```python
from build123d import *

# Parameters (mm, degrees)
SKETCH_4_R      = 1
EXTRUDE_1_DEPTH = 3


with BuildPart() as part:
    # ｽｹｯﾁ4 → ﾎﾞｽ - 押し出し1 (new body)
    with BuildSketch(Plane(origin=(0, 0, 0), x_dir=(1, 0, 0), z_dir=(0, 1, 0))):
        with BuildLine():
            Line((13.643014387, 25.949889929), (-16.356985613, 25.949889929))
            ThreePointArc((-16.356985613, 25.949889929), (-23.428053425, 23.020957741), (-26.356985613, 15.949889929))
            Line((-26.356985613, 15.949889929), (-26.356985613, -14.050110071))
            ThreePointArc((-26.356985613, -14.050110071), (-23.428053425, -21.121177883), (-16.356985613, -24.050110071))
            Line((-16.356985613, -24.050110071), (13.643014387, -24.050110071))
            ThreePointArc((13.643014387, -24.050110071), (20.714082199, -21.121177883), (23.643014387, -14.050110071))
            Line((23.643014387, -14.050110071), (23.643014387, 15.949889929))
            ThreePointArc((23.643014387, 15.949889929), (20.714082199, 23.020957741), (13.643014387, 25.949889929))
        make_face()
        with Locations(Location((16.643014387, -17.050110071, 0), (0, 0, 270))):
            Circle(SKETCH_4_R, mode=Mode.SUBTRACT)
        with Locations(Location((16.643014387, 18.949889929, 0), (0, 0, 270))):
            Circle(SKETCH_4_R, mode=Mode.SUBTRACT)
        with Locations(Location((-19.356985613, 18.949889929, 0), (0, 0, 270))):
            Circle(SKETCH_4_R, mode=Mode.SUBTRACT)
        with Locations(Location((-19.356985613, -17.050110071, 0), (0, 0, 270))):
            Circle(SKETCH_4_R, mode=Mode.SUBTRACT)
        with Locations(Location((-1.356985613, 0.949889929, 0), (0, 0, 270))):
            Circle(SKETCH_4_R, mode=Mode.SUBTRACT)
    extrude(amount=EXTRUDE_1_DEPTH)


solid = part.part
```
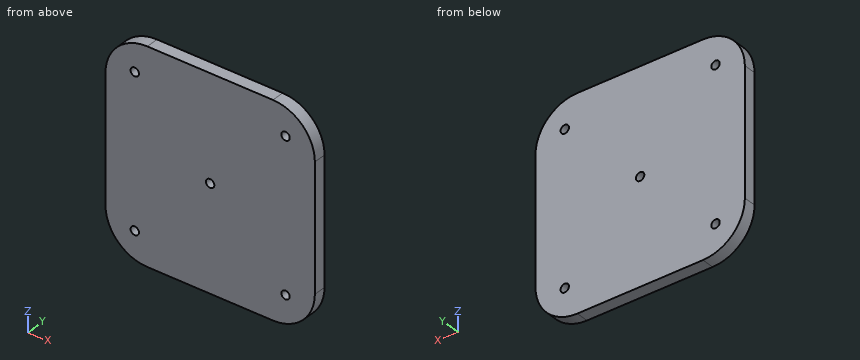
Can you work these out from the model? Positions are in its coordinate system, mm. Coordinates: 2 decimals unless noted, no trailing zeros. Order: outer loops, then holes, each group sorted by start corner. A loop starts at its lowest first (then second) coordinate and runs counter-clockwise, first axis right, second up. Notation, with made-up numbers: (-38, 84.5) - (-28, 84.5) arc R10 cw to (-28, 90.5) - close; hole circle Ø2 at (-26, -34.5). An arc over 180 degrees is marked (long way). Answer in a Markdown table with one row per item.
1. For pin 1 (10 mm diameter, centred on x = 17.5, z = 5, fed in from -Y), with a flat end and sliding along its axis, tell me the tip position at first contact or that it passes through.
Reply:
| item | result |
|---|---|
| pin 1 | stops at y = 0 |
2. Suppose I cut it at C-C (z = 20.5). Please give me the cut outline in (x, y), and give its area (3 significant figures).
Reply:
| item | result |
|---|---|
| outline | (-24, 0) - (21.28, 0) - (21.28, 3) - (-24, 3) - close |
| area | 136 mm^2 |
3. Suppose I cut it at A-A (y = 1.7). Please give me the cut outline in (x, z).
Reply:
| item | result |
|---|---|
| outline | (-26.36, -15.95) arc R10 ccw to (-16.36, -25.95) - (13.64, -25.95) arc R10 ccw to (23.64, -15.95) - (23.64, 14.05) arc R10 ccw to (13.64, 24.05) - (-16.36, 24.05) arc R10 ccw to (-26.36, 14.05) - close; hole circle Ø2 at (-19.36, -18.95); hole circle Ø2 at (-19.36, 17.05); hole circle Ø2 at (-1.36, -0.95); hole circle Ø2 at (16.64, -18.95); hole circle Ø2 at (16.64, 17.05) |
4. If I drill on line 1 along Z through (x, y) = (-2, 2.7); line 2 along X through (y, z) = (1.1, -0.5); line 3 along X through (y, z) = (0.2, 15), over which ranges is the centre line in solid material (lowest first)?
Reply:
| item | result |
|---|---|
| line 1 | z = -25.95 to -1.72, -0.18 to 24.05 |
| line 2 | x = -26.36 to -2.25, -0.46 to 23.64 |
| line 3 | x = -26.31 to 23.6 |
5. Suppose I cut it at B-B (x = 21). Please give me the cut outline in (y, z).
Reply:
| item | result |
|---|---|
| outline | (0, -22.72) - (3, -22.72) - (3, 20.82) - (0, 20.82) - close |
